```python
from build123d import *

# Parameters (mm, degrees)
F1_DEPTH = 25.4


with BuildPart() as f1:
    # F0 (on Front) → F1 (new body)
    with BuildSketch(Plane.XZ):
        Polygon((10, 21.561685), (-10, 50), (-10, -50), (10, -50), align=None)
        Polygon((10, 50), (-10, 50), (10, 21.561685), align=None)
        Polygon((33.010388, 17.281167), (10, 50), (10, 21.561685), (13.010388, 17.281167), align=None)
    extrude(amount=F1_DEPTH)


solid = f1.part
```
Geometry: final body of the model. Coordinates: model frame, mm. A direction names the side the tool comes from. Give positions to 0.01 mm unless a question says otherwise; leave off trailing zeros. Order: outer loops, then holes, each group sorted by start corner. A loop starts at its lowest first (then second) coordinate and runs counter-clockwise, first axis right, second up. Notation, with made-up numbers: M -18,63.5 L 25,63.5 A13 cw 25,88.5 Z; hole C 35.25,26 d3. An arc over 180 degrees is marked long. Answer as CSV lines item,"result". Start each with the question number.
1) Cut plane B-B (z = -11). Output: boundary loops of the cut face in (x, y), then the cut area to 3 significant figures.
2) Mould query, pull axis X, two halves, no side actions, for faces 1 (the flat face through (11.484, -12.522, 19.451)), 2 (the flat face through (-10, -13, 1)), 3 (the flat face through (0, -13, -50)). Classes: +X half, -X half, draft (parallel to the pull), parting line (faces both ways), or undercut.
3) Line query: line 1 (X direction, y = -14, z = 4); line 2 (X direction, y = -7, z = 18); line 3 (X direction, y = -20.5, z = 27.5). Output: solid intervals per line, ascending. Write a range as from..to.
4) Cut plane A-A (y = -4.25). Output: boundary loops of the cut face in (x, z), then the cut area to 3 significant figures.
5) Set-up query: faces 4 (the flat face through (2, -25.4, 1)), 5 (the flat face through (23, -13, 17.281)). Return all of +Z, -Z, +X, -X, +Y, -Y with unobstructed straight access to the full face (end or side cutting, diameter ignored); none if empty.
6) First-contact query: P1, Ø8, axis at x = -2.5, z = 9, coming from the +Y side; P2, Ø1, axis at x = 13.5, y = -7.5, coming from the +Z side; P3, Ø2, axis at y = -6.5, z = -28, coming from the +X side; P4, Ø1.5, axis at x = 21.5, y = -19, coming from the +Z side. Flat tips, straight axial feed; report the tip coordinate or a pass-through.
7) Cut plane C-C (x = 25.5). Output: boundary loops of the cut face in (y, z), then the cut area to 3 significant figures.
Findings below:
1,outline,"M -10,-25.4 L 10,-25.4 L 10,0 L -10,0 Z"
1,area,"508 mm²"
2,face 1,"undercut"
2,face 2,"-X half"
2,face 3,"draft"
3,line 1,"x = -10..10"
3,line 2,"x = -10..10, 12.5..32.5"
3,line 3,"x = -10..25.82"
4,outline,"M -10,-50 L 10,-50 L 10,21.56 L 13.01,17.28 L 33.01,17.28 L 10,50 L -10,50 Z"
4,area,"2,370 mm²"
5,face 4,"+Z, -Z, +X, -X, -Y"
5,face 5,"-Z, +X, +Y, -Y"
6,P1,"stops at y = 0"
6,P2,"stops at z = 45.73"
6,P3,"stops at x = 10"
6,P4,"stops at z = 34.71"
7,outline,"M -25.4,17.28 L 0,17.28 L 0,27.96 L -25.4,27.96 Z"
7,area,"271 mm²"
